Read the model definition and answer for the solid it produces. Units are mm, in the model's axes. A direction names the side the tool comes from. Coordinates: 2 decimals unless noted, no trailing zeros. Loops run counter-clockwise (first coordinate to the right, second up) from the corner with the lowest first, then second, coordinate; pieces in that order, holes last. Notation, with made-up numbers: (-5.75, 40.25) - (35.25, 40.25) arc R22 cw to (35.25, 75.25) - close; hole circle Ø7 at (54, 63). An arc over 180 degrees is marked (long way). One line per question, with ' | ' between items. Start each with the question number.
```python
from build123d import *

# Parameters (mm, degrees)
SALIENTE_EXTRUIR1_DEPTH = 25
SALIENTE_EXTRUIR2_DEPTH = 15
SALIENTE_EXTRUIR3_START = -25
SALIENTE_EXTRUIR3_DEPTH = 20


with BuildPart() as part:
    # Croquis1 → Saliente-Extruir1 (new, symmetric)
    with BuildSketch(Plane(origin=(0, 0, 0), x_dir=(0, 0, -1), z_dir=(1, 0, 0))):
        Polygon((29, -27.5), (39, -27.5), (39, 27.5), (-39, 27.5), (-39, -27.5), (-29, -27.5), (-29, 4.5), (29, 4.5), align=None)
    extrude(amount=SALIENTE_EXTRUIR1_DEPTH, both=True)

    # Croquis2 → Saliente-Extruir2 (add, symmetric)
    with BuildSketch(Plane(origin=(0, 0, 0), x_dir=(0, 0, -1), z_dir=(1, 0, 0))):
        Polygon((-26, 27.5), (-26, 37.5), (-42.5, 37.5), (-57, -7.5), (-57, -27.5), (-39, -27.5), (-39, 27.5), align=None)
        Polygon((39, -27.5), (39, 27.5), (26, 27.5), (26, 37.5), (42.5, 37.5), (57, -7.5), (57, -27.5), align=None)
    extrude(amount=SALIENTE_EXTRUIR2_DEPTH, both=True)

    # Croquis3 → Saliente-Extruir3 (add)
    with BuildSketch(Plane(origin=(0, 0, 0), x_dir=(0, 0, -1), z_dir=(1, 0, 0)).offset(SALIENTE_EXTRUIR3_START)):
        with BuildLine():
            Line((-20, 27.5), (20, 27.5))
            ThreePointArc((20, 27.5), (0, 47.5), (-20, 27.5))
        make_face()
    extrude(amount=SALIENTE_EXTRUIR3_DEPTH)


solid = part.part
```
1) The part is cut by section D-D on y = 24.5. Write down the section's boundary in (x, z).
2) The mould has two halves that part along Z. Classify faces 1 (the flat face through (-0.21, 15.31, 49.65)), 2 (the flat face through (0, 32, -26)), 3 (the flat face through (0, -27.5, 40)), 4 (the flat face through (0.21, 15.31, -49.65)): released by +Z, released by -Z, zero draft, split by the parting line, or undercut.
3) Which of the six approach directions +Z, -Z, +X, -X, +Y, -Y give full straight-line access (tool end or side, diameter ignored) to faces 5 (the flat face through (-5, 35, 0)), 6 (the flat face through (20, 0, 39)), 7 (the flat face through (0, -11, -29))?
4) The part is cut by section B-B on x = 10. Write down the section's boundary in (y, z).
5) Given pin 1 Ø4 at (x, y) = (4.5, 8) entering from +Z; pin 2 Ø18 at (x, z) = (-7, -36.5) entering from +Y; pin 3 Ø8 at (y, z) = (19, -43.5) entering from -X; pin 4 Ø1 at (y, z) = (2.5, -26) entering from -X, each flat-ended and moving along its own axis, determine where each tip first touches the part or whether it passes through.
6) The part is cut by section A-A on y = -9. Write down the section's boundary in (x, z).
7) Find the intervals of material crossed by line 1 along Z through (x, y) = (-1, -24); line 2 along Z through (x, y) = (23, -17.5); line 3 along Y through (x, z) = (8, -10.5), in increasing order. Write a range as from..to.
8) The part is cut by section C-C on z = 0. Write down the section's boundary in (x, y), and give its area (3 significant figures).
Answer below:
1) outline: (-25, -39) - (-15, -39) - (-15, -46.69) - (15, -46.69) - (15, -39) - (25, -39) - (25, 39) - (15, 39) - (15, 46.69) - (-15, 46.69) - (-15, 39) - (-25, 39) - close
2) face 1: released by +Z | face 2: undercut | face 3: zero draft | face 4: released by -Z
3) face 5: +X, +Y | face 6: +Z, +X, +Y, -Y | face 7: +X, -X, -Y
4) outline: (-27.5, -57) - (-7.5, -57) - (37.5, -42.5) - (37.5, -26) - (27.5, -26) - (27.5, 26) - (37.5, 26) - (37.5, 42.5) - (-7.5, 57) - (-27.5, 57) - (-27.5, 29) - (4.5, 29) - (4.5, -29) - (-27.5, -29) - close
5) pin 1: z = 52.65 | pin 2: y = 37.5 | pin 3: x = -15 | pin 4: through
6) outline: (-25, -39) - (-15, -39) - (-15, -57) - (15, -57) - (15, -39) - (25, -39) - (25, -29) - (-25, -29) - close; (-25, 29) - (25, 29) - (25, 39) - (15, 39) - (15, 57) - (-15, 57) - (-15, 39) - (-25, 39) - close
7) line 1: -57..-29, 29..57 | line 2: -39..-29, 29..39 | line 3: 4.5..27.5
8) outline: (-25, 4.5) - (25, 4.5) - (25, 27.5) - (-5, 27.5) - (-5, 47.5) - (-25, 47.5) - close | area: 1,550 mm2
